```python
from build123d import *

# Parameters (mm, degrees)
F0_W      = 127
F0_H      = 38.1
F1_DEPTH  = 63.5
F2_W      = 9.525
F2_H      = 12.7
F3_DEPTH  = 127.001
F4_W      = 9.525
F4_H      = 12.7
F5_DEPTH  = 127.001
F6_R      = 9.525
F7_DEPTH  = 127.001
F8_R      = 9.525
F9_DEPTH  = 38.101
F10_R     = 9.525
F11_DEPTH = 38.101


with BuildPart() as f1:
    # F0 (on Top) → F1 (new body)
    with BuildSketch(Plane.XY):
        with Locations((-20.138042, -12.861965)):
            Rectangle(F0_W, F0_H)
    extrude(amount=F1_DEPTH)

    # F2 (on face) → F3 (cut, through all)
    with BuildSketch(Plane.YZ.offset(43.361958)):
        with Locations((-27.149465, 6.35)):
            Rectangle(F2_W, F2_H)
    extrude(amount=-F3_DEPTH, mode=Mode.SUBTRACT)

    # F4 (on face) → F5 (cut, through all)
    with BuildSketch(Plane.YZ.offset(43.361958)):
        with Locations((1.425535, 6.35)):
            Rectangle(F4_W, F4_H)
    extrude(amount=-F5_DEPTH, mode=Mode.SUBTRACT)

    # F6 (on face) → F7 (cut, through all)
    with BuildSketch(Plane.YZ.offset(43.361958)):
        with Locations((-12.861965, 38.1)):
            Circle(F6_R)
    extrude(amount=-F7_DEPTH, mode=Mode.SUBTRACT)

    # F8 (on face) → F9 (cut, through all)
    with BuildSketch(Plane.XZ.offset(31.911965)):
        with Locations((-51.888042, 38.1)):
            Circle(F8_R)
    extrude(amount=-F9_DEPTH, mode=Mode.SUBTRACT)

    # F10 (on face) → F11 (cut, through all)
    with BuildSketch(Plane.XZ.offset(31.911965)):
        with Locations((11.611958, 38.1)):
            Circle(F10_R)
    extrude(amount=-F11_DEPTH, mode=Mode.SUBTRACT)


solid = f1.part
```
Source: CAD feature listing. Evaluate the final solid. Frame: model axes, mm. A direction names the side the tool comes from. Coordinates: 2 decimals unless noted, no trailing zeros. Order: outer loops, then holes, each group sorted by start corner. A loop starts at its lowest first (then second) coordinate and runs counter-clockwise, first axis right, second up. Notation, with made-up numbers: M -22,-5 L 32,-5 A26 cw 32,21 Z; hole C -11.75,66.5 d7. An arc over 180 degrees is marked long. Write each question's results on one line, items separated by ' | '. Start each with the question number.
1) Line query: line 1 (X direction, y = 0, z = 38); line 2 (Y direction, x = -67, z = 38.1); line 3 (Z direction, x = 4, y = -1). Output: solid intervals per line, ascending. Write a range as from..to.
2) Section query B-B (x = -45). Return the cut outline in (y, z) (3 decimals).
3) Section query A-A (z = 38.1). Return the cut outline in (x, y).
4) Contact query for flat-ended pins moving along their axis: pin 1 Ø4 at (x, z) = (-43, 9) entering from -Y; pin 2 Ø5 at (x, y) = (-47, -25) entering from -Z. Output: stop coordinate, or through.
5) Draft query along X for faces 1 (the face through (-42.803, -1.354, 40.961)), 2 (the face through (-46.767, -24.637, 46.132)), 3 (the face through (-83.638, -5, 31)), 4 (the face through (-19, -3.337, 6)). Return one class per face: released by +X, released by -X, zero draft, split by the parting line, or undercut.
6) Access query for faces 5 (the face through (-19, -27, 12.7)), 6 (the face through (20.697, -1.354, 40.961)), 7 (the face through (-19, 1, 12.7)). Directions: +Z, -Z, +X, -X, +Y, -Y. A direction counts if a zero-diameter tool reaches every point of the face in a straight line with its end or side. Return the directions, or none.
7) Section query C-C (y = -6.5). Return the cut outline in (x, z) (3 decimals).
8) Section query D-D (z = 8). Return the cut outline in (x, y), plus the area to 3 significant figures.
Answers:
1) line 1: x = -83.64..-61.41, -42.36..2.09, 21.14..43.36 | line 2: y = -31.91..-22.39, -3.34..6.19 | line 3: z = 12.7..32.37, 43.83..63.5
2) outline: M -31.912,12.7 L -22.387,12.7 L -22.387,0 L -3.337,0 L -3.337,12.7 L 6.188,12.7 L 6.188,31.521 L -5.974,31.521 A9.525 cw -19.75,31.521 L -31.912,31.521 Z; M -31.912,44.679 L -19.75,44.679 A9.525 cw -5.974,44.679 L 6.188,44.679 L 6.188,63.5 L -31.912,63.5 Z
3) outline: M -83.64,-31.91 L -61.41,-31.91 L -61.41,-22.39 L -83.64,-22.39 Z; M -83.64,-3.34 L -61.41,-3.34 L -61.41,6.19 L -83.64,6.19 Z; M -42.36,-31.91 L 2.09,-31.91 L 2.09,-22.39 L -42.36,-22.39 Z; M -42.36,-3.34 L 2.09,-3.34 L 2.09,6.19 L -42.36,6.19 Z; M 21.14,-31.91 L 43.36,-31.91 L 43.36,-22.39 L 21.14,-22.39 Z; M 21.14,-3.34 L 43.36,-3.34 L 43.36,6.19 L 21.14,6.19 Z
4) pin 1: stops at y = -22.39 | pin 2: stops at z = 12.7
5) face 1: undercut | face 2: undercut | face 3: released by -X | face 4: zero draft
6) face 5: -Z, +X, -X, -Y | face 6: +Y, -Y | face 7: -Z, +X, -X, +Y
7) outline: M -83.638,0 L 43.362,0 L 43.362,31.011 L 17.974,31.011 A9.525 cw 5.25,31.011 L -45.526,31.011 A9.525 cw -58.25,31.011 L -83.638,31.011 Z; M -83.638,45.189 L -58.25,45.189 A9.525 cw -45.526,45.189 L 5.25,45.189 A9.525 cw 17.974,45.189 L 43.362,45.189 L 43.362,63.5 L -83.638,63.5 Z
8) outline: M -83.64,-22.39 L 43.36,-22.39 L 43.36,-3.34 L -83.64,-3.34 Z | area: 2,420 mm^2
